```python
from build123d import *

# Parameters (mm, degrees)
SKETCH2_W                      = 45
SKETCH2_H                      = 24
BOSS_EXTRUDE1_DEPTH            = 50
CUT_EXTRUDE7_DEPTH             = 50
CHAMFER4_SIZE                  = 6
CUT_EXTRUDE1_REACH             = 70.33
SKETCH3_W                      = 45
SKETCH3_H                      = 10
CUT_EXTRUDE2_REACH             = 55.912
SKETCH4_R                      = 2
CUT_EXTRUDE2_DIRECTION_2_REACH = 55.912
SKETCH8_W                      = 45
SKETCH8_H                      = 50
CUT_EXTRUDE4_DEPTH             = 14
SKETCH6_R                      = 4
BOSS_EXTRUDE2_DEPTH            = 45
CUT_EXTRUDE3_START             = -50
SKETCH7_R                      = 2
CUT_EXTRUDE3_DEPTH             = 50
CUT_EXTRUDE6_START             = -2.5
SKETCH13_R                     = 2
CUT_EXTRUDE6_DEPTH             = 50
BOSS_EXTRUDE16_REACH           = 58.127
CUT_EXTRUDE13_REACH            = 64.292
SKETCH30_W                     = 45
SKETCH30_H                     = 10
CUT_EXTRUDE18_START            = -50
SKETCH37_R                     = 2
CUT_EXTRUDE18_DEPTH            = 50
CUT_EXTRUDE20_REACH            = 62.83
SKETCH43_R                     = 1.5
SKETCH44_R                     = 3.05
CUT_EXTRUDE21_DEPTH            = 1.1
SKETCH45_R                     = 3.05
CUT_EXTRUDE22_DEPTH            = 1.1
BOSS_EXTRUDE23_DEPTH           = 2.5
BOSS_EXTRUDE24_DEPTH           = 2.5
SKETCH55_R                     = 3.05
CUT_EXTRUDE28_DEPTH            = 1.1
CUT_EXTRUDE29_START            = -50
SKETCH57_R                     = 1.5
CUT_EXTRUDE29_DEPTH            = 48.9
SKETCH58_R                     = 3.05
CUT_EXTRUDE30_DEPTH            = 1.1
CHAMFER11_SIZE                 = 3
BOSS_EXTRUDE19_DEPTH           = 8
BOSS_EXTRUDE20_DEPTH           = 8
CHAMFER7_SIZE                  = 1
CHAMFER8_SIZE                  = 1


with BuildPart() as part:
    # Sketch2 → Boss-Extrude1 (new body)
    with BuildSketch(Plane(origin=(0, 0, 0), x_dir=(0, 0, -1), z_dir=(1, 0, 0))):
        Rectangle(SKETCH2_W, SKETCH2_H)
    extrude(amount=BOSS_EXTRUDE1_DEPTH)

    # Sketch14 → Cut-Extrude7 (cut)
    with BuildSketch(Plane(origin=(50, 0, 0), x_dir=(0, 0, -1), z_dir=(1, 0, 0))):
        Polygon((2.5, 12), (22.5, 2), (22.5, 12), align=None)
    extrude(amount=-CUT_EXTRUDE7_DEPTH, mode=Mode.SUBTRACT)

    # Chamfer4
    chamfer4_edges = [part.edges().sort_by_distance(p)[0] for p in [
        (25, -12, 22.5),
        (25, 12, 22.5),
    ]]
    chamfer(chamfer4_edges, length=CHAMFER4_SIZE)

    # Cut-Extrude1: up to this face of the body (flat: up to its plane)
    cut_extrude1_end = Plane(part.part.faces().sort_by_distance((25, 0, 22.5))[0])
    # Sketch3 → Cut-Extrude1 (cut, up to the picked face)
    with BuildSketch(Plane(origin=(0, 0, -22.5), x_dir=(-1, 0, 0), z_dir=(0, 0, -1)), mode=Mode.PRIVATE) as cut_extrude1_sk1:
        with Locations((-25, -7)):
            Rectangle(SKETCH3_W, SKETCH3_H)
    cut_extrude1_tool1 = split(extrude(cut_extrude1_sk1.sketch, amount=-CUT_EXTRUDE1_REACH, mode=Mode.PRIVATE), bisect_by=cut_extrude1_end, keep=Keep.BOTH, mode=Mode.PRIVATE)
    add(cut_extrude1_tool1.solids().sort_by(Axis((25, -7, -22.5), (0, 0, 1)))[0], mode=Mode.SUBTRACT)

    # Cut-Extrude2: up to this face of the body (flat: up to its plane)
    cut_extrude2_end = Plane(part.part.faces().sort_by_distance((50, -0.918079096, 0.895480226))[0])
    # Sketch4 → Cut-Extrude2 (cut, up to the picked face)
    with BuildSketch(Plane(origin=(2.5, 0, 0), x_dir=(0, 0, -1), z_dir=(1, 0, 0)), mode=Mode.PRIVATE) as cut_extrude2_sk1:
        with Locations(Location((14.5, -4, 0), (0, 0, 180))):
            Circle(SKETCH4_R)
    cut_extrude2_tool1 = split(extrude(cut_extrude2_sk1.sketch, amount=CUT_EXTRUDE2_REACH, mode=Mode.PRIVATE), bisect_by=cut_extrude2_end, keep=Keep.BOTH, mode=Mode.PRIVATE)
    add(cut_extrude2_tool1.solids().sort_by(Axis((2.5, -4, -14.5), (1, 0, 0)))[0], mode=Mode.SUBTRACT)

    # Cut-Extrude2 direction 2: up to this face of the body (flat: up to its plane)
    cut_extrude2_direction_2_end = Plane(part.part.faces().sort_by_distance((0, -0.918079096, 0.895480226))[0])
    # Sketch4 → Cut-Extrude2 direction 2 (cut, up to the picked face)
    with BuildSketch(Plane(origin=(2.5, 0, 0), x_dir=(0, 0, -1), z_dir=(1, 0, 0)), mode=Mode.PRIVATE) as cut_extrude2_direction_2_sk1:
        with Locations(Location((14.5, -4, 0), (0, 0, 180))):
            Circle(SKETCH4_R)
    cut_extrude2_direction_2_tool1 = split(extrude(cut_extrude2_direction_2_sk1.sketch, amount=-CUT_EXTRUDE2_DIRECTION_2_REACH, mode=Mode.PRIVATE), bisect_by=cut_extrude2_direction_2_end, keep=Keep.BOTH, mode=Mode.PRIVATE)
    add(cut_extrude2_direction_2_tool1.solids().sort_by(Axis((2.5, -4, -14.5), (-1, 0, 0)))[0], mode=Mode.SUBTRACT)

    # Sketch8 → Cut-Extrude4 (cut)
    with BuildSketch(Plane(origin=(0, 12, 0), x_dir=(1, 0, 0), z_dir=(0, 1, 0))):
        with Locations((25, 2.5)):
            Rectangle(SKETCH8_W, SKETCH8_H)
    extrude(amount=-CUT_EXTRUDE4_DEPTH, mode=Mode.SUBTRACT)


with BuildPart() as cut_extrude4_piece_1:
    # of the separate pieces the step leaves, piece 1, a body of its own (cut_extrude4_pieces)
    add(part.part.solids().sort_by_distance((0, -12, 16.5))[0])


with BuildPart() as cut_extrude4_piece_2:
    # of the separate pieces the step leaves, piece 2, a body of its own (cut_extrude4_pieces)
    add(part.part.solids().sort_by_distance((50, 2, -22.5))[0])

    # Sketch6 → Boss-Extrude2 (add)
    with BuildSketch(Plane(origin=(2.5, 0, 0), x_dir=(0, 0, -1), z_dir=(1, 0, 0))):
        with Locations(Location((14.5, -4, 0), (0, 0, 180))):
            Circle(SKETCH6_R)
    extrude(amount=BOSS_EXTRUDE2_DEPTH)


with BuildPart() as cut_extrude3_tool:
    # Sketch7 → Cut-Extrude3 (new body)
    with BuildSketch(Plane.ZY.offset(CUT_EXTRUDE3_START)):
        with Locations((11, 0)):
            Circle(SKETCH7_R)
    extrude(amount=CUT_EXTRUDE3_DEPTH)


with BuildPart() as cut_extrude4_piece_1_1:
    add(cut_extrude4_piece_1.part)

    # Cut-Extrude3: cut by cut_extrude3_tool
    add(cut_extrude3_tool.part, mode=Mode.SUBTRACT)


with BuildPart() as cut_extrude4_piece_2_1:
    add(cut_extrude4_piece_2.part)

    # Cut-Extrude3: cut by cut_extrude3_tool
    add(cut_extrude3_tool.part, mode=Mode.SUBTRACT)


with BuildPart() as cut_extrude6_tool:
    # Sketch13 → Cut-Extrude6 (new body)
    with BuildSketch(Plane.ZY.offset(-47.5).offset(CUT_EXTRUDE6_START)):
        with Locations(Location((-2.5, -4, 0), (0, 0, 270))):
            Circle(SKETCH13_R)
    extrude(amount=CUT_EXTRUDE6_DEPTH)


with BuildPart() as cut_extrude4_piece_1_2:
    add(cut_extrude4_piece_1_1.part)

    # Cut-Extrude6: cut by cut_extrude6_tool
    add(cut_extrude6_tool.part, mode=Mode.SUBTRACT)


with BuildPart() as cut_extrude4_piece_2_2:
    add(cut_extrude4_piece_2_1.part)

    # Cut-Extrude6: cut by cut_extrude6_tool
    add(cut_extrude6_tool.part, mode=Mode.SUBTRACT)

    # Boss-Extrude16: up to this face of the body (flat: up to its plane)
    boss_extrude16_end = Plane(cut_extrude4_piece_2_2.part.faces().sort_by_distance((50, -0.845343651, 1.015922603))[0])
    # Sketch29 → Boss-Extrude16 (add, up to the picked face)
    with BuildSketch(Plane.ZY, mode=Mode.PRIVATE) as boss_extrude16_sk1:
        Polygon((28.985281374, 6), (22.5, 6), (22.5, -6), (28.985281374, -6), (32.5, -2.485281374), (32.5, 2.485281374), align=None)
    boss_extrude16_tool1 = split(extrude(boss_extrude16_sk1.sketch, amount=-BOSS_EXTRUDE16_REACH, mode=Mode.PRIVATE), bisect_by=boss_extrude16_end, keep=Keep.BOTH, mode=Mode.PRIVATE)

    add(cut_extrude4_piece_1_2.part)  # Boss-Extrude16 merges Cut-Extrude4 piece 1
    add(boss_extrude16_tool1.solids().sort_by(Axis((0, 0, 27.06066), (1, 0, 0)))[0])

    # Cut-Extrude13: up to this plane
    cut_extrude13_end = Plane(origin=(65.620499352, -6, 28.985281374), z_dir=(0, -0.7071067811865474, 0.7071067811865477))
    # Sketch30 → Cut-Extrude13 (cut, up to the surface)
    with BuildSketch(Plane(origin=(0, 6, 0), x_dir=(1, 0, 0), z_dir=(0, 1, 0)), mode=Mode.PRIVATE) as cut_extrude13_sk1:
        with Locations((25, -27.5)):
            Rectangle(SKETCH30_W, SKETCH30_H)
    cut_extrude13_tool1 = split(extrude(cut_extrude13_sk1.sketch, amount=-CUT_EXTRUDE13_REACH, mode=Mode.PRIVATE), bisect_by=cut_extrude13_end, keep=Keep.BOTH, mode=Mode.PRIVATE)
    add(cut_extrude13_tool1.solids().sort_by_distance((25, 6, 27.5))[0], mode=Mode.SUBTRACT)

    # Sketch37 → Cut-Extrude18 (cut)
    with BuildSketch(Plane.ZY.offset(CUT_EXTRUDE18_START)):
        with Locations((27.5, 0)):
            Circle(SKETCH37_R)
    extrude(amount=CUT_EXTRUDE18_DEPTH, mode=Mode.SUBTRACT)

    # Cut-Extrude20: up to this face of the body (flat: up to its plane)
    cut_extrude20_end = Plane(cut_extrude4_piece_2_2.part.faces().sort_by_distance((0, -0.765078921, 3.483337135))[0])
    # Sketch43 → Cut-Extrude20 (cut, up to the picked face)
    with BuildSketch(Plane(origin=(50, 0, 0), x_dir=(0, 0, -1), z_dir=(1, 0, 0)), mode=Mode.PRIVATE) as cut_extrude20_sk1:
        with Locations((7.5, 3)):
            Circle(SKETCH43_R)
    cut_extrude20_tool1 = split(extrude(cut_extrude20_sk1.sketch, amount=-CUT_EXTRUDE20_REACH, mode=Mode.PRIVATE), bisect_by=cut_extrude20_end, keep=Keep.BOTH, mode=Mode.PRIVATE)
    add(cut_extrude20_tool1.solids().sort_by(Axis((50, 3, -7.5), (-1, 0, 0)))[0], mode=Mode.SUBTRACT)

    # Sketch44 → Cut-Extrude21 (cut)
    with BuildSketch(Plane(origin=(50, 0, 0), x_dir=(0, 0, -1), z_dir=(1, 0, 0))):
        with Locations((7.5, 3)):
            Circle(SKETCH44_R)
    extrude(amount=-CUT_EXTRUDE21_DEPTH, mode=Mode.SUBTRACT)

    # Sketch45 → Cut-Extrude22 (cut)
    with BuildSketch(Plane.ZY):
        with Locations(Location((-7.5, 3, 0), (0, 0, 180))):
            Circle(SKETCH45_R)
    extrude(amount=-CUT_EXTRUDE22_DEPTH, mode=Mode.SUBTRACT)

    # Sketch48 → Boss-Extrude23 (add)
    with BuildSketch(Plane(origin=(50, 0, 0), x_dir=(0, 0, -1), z_dir=(1, 0, 0))):
        Polygon((-16.5, 12), (-22.5, 6), (-28.985281374, 6), (-32.5, 2.485281374), (-32.5, 12), align=None)
    extrude(amount=-BOSS_EXTRUDE23_DEPTH)

    # Sketch49 → Boss-Extrude24 (add)
    with BuildSketch(Plane.ZY):
        Polygon((28.985281374, 6), (22.5, 6), (16.5, 12), (32.5, 12), (32.5, 2.485281374), align=None)
    extrude(amount=-BOSS_EXTRUDE24_DEPTH)

    # Sketch55 → Cut-Extrude28 (cut)
    with BuildSketch(Plane.ZY):
        with Locations((27.5, 7)):
            Circle(SKETCH55_R)
    extrude(amount=-CUT_EXTRUDE28_DEPTH, mode=Mode.SUBTRACT)

    # Sketch57 → Cut-Extrude29 (cut)
    with BuildSketch(Plane.ZY.offset(CUT_EXTRUDE29_START)):
        with Locations((27.5, 7)):
            Circle(SKETCH57_R)
    extrude(amount=CUT_EXTRUDE29_DEPTH, mode=Mode.SUBTRACT)

    # Sketch58 → Cut-Extrude30 (cut)
    with BuildSketch(Plane(origin=(50, 0, 0), x_dir=(0, 0, -1), z_dir=(1, 0, 0))):
        with Locations(Location((-27.5, 7, 0), (0, 0, 180))):
            Circle(SKETCH58_R)
    extrude(amount=-CUT_EXTRUDE30_DEPTH, mode=Mode.SUBTRACT)

    # Chamfer11
    chamfer11_edges = [cut_extrude4_piece_2_2.edges().sort_by_distance(p)[0] for p in [
        (48.75, 12, 32.5),
        (1.25, 12, 32.5),
    ]]
    chamfer(chamfer11_edges, length=CHAMFER11_SIZE)

    # Sketch38 → Boss-Extrude19 (add)
    with BuildSketch(Plane.ZY):
        Polygon((-2.5, 12), (-22.5, 2), (-22.5, -12), (16.5, -12), (22.5, -6), (22.5, 6), (16.5, 12), align=None)
    extrude(amount=BOSS_EXTRUDE19_DEPTH)

    # Sketch39 → Boss-Extrude20 (add)
    with BuildSketch(Plane(origin=(50, 0, 0), x_dir=(0, 0, -1), z_dir=(1, 0, 0))):
        Polygon((-22.5, 6), (-22.5, -6), (-16.5, -12), (22.5, -12), (22.5, 2), (2.5, 12), (-16.5, 12), align=None)
    extrude(amount=BOSS_EXTRUDE20_DEPTH)

    # Chamfer7
    chamfer7_edges = [cut_extrude4_piece_2_2.edges().sort_by_distance(p)[0] for p in [
        (-8, 12, 7),
        (-8, 7, -12.5),
        (-8, -5, -22.5),
        (-8, -12, -3),
        (-8, -9, 19.5),
        (-8, 0, 22.5),
        (-8, 9, 19.5),
        (58, 9, 19.5),
        (58, 0, 22.5),
        (58, -9, 19.5),
        (58, -12, -3),
        (58, -5, -22.5),
        (58, 7, -12.5),
        (58, 12, 7),
    ]]
    chamfer(chamfer7_edges, length=CHAMFER7_SIZE)

    # Chamfer8
    chamfer8_edges = [cut_extrude4_piece_2_2.edges().sort_by_distance(p)[0] for p in [
        (47.5, -12, -3),
        (47.5, -5, -22.5),
        (47.5, -9, 19.5),
        (47.5, 7, -12.5),
    ]]
    chamfer(chamfer8_edges, length=CHAMFER8_SIZE)


solid = cut_extrude4_piece_2_2.part
```
Model file for the job. Use its own axes, mm. A direction names the side the tool comes from. Coordinates: 2 decimals unless noted, no trailing zeros. Order: outer loops, then holes, each group sorted by start corner. A loop starts at its lowest first (then second) coordinate and runs counter-clockwise, first axis right, second up. Notation, with made-up numbers: (71.5, -32) -> (90.5, -32) arc R21 ccw to (90.5, -1) -> close; hole circle Ø9 at (23.5, -12). An arc over 180 degrees is marked (long way). Answer as a JSON object with one key per item and string values. Group by question number.
1) Drill centre lines: L1, parallel to X at y = 11.25, z = 20.5; L2, parallel to Y at x = 1.7, z = -2.5; L3, parallel to X at y = -2.5, z = 7. Where is each one in solid material? Low to high.
2) Flat gauge pins, fed straight in: pin 1 (3 mm diameter, centred on y = 0, z = 27.5, fed in from +X); pin 2 (13 mm diameter, centred on y = 4.5, z = 23, fed in from -X); pin 3 (4 mm diameter, centred on y = 7, z = 27.5, fed in from -X); pin 4 (2 mm diameter, centred on x = 52.5, y = 1, fed in from +Z). Where does each tip first touch, or does it go through?
3) Cut at A-A, the plane z = 11. Write the cut outline in (x, y).
4) Cut at B-B, the plane y = 7. Count the separate pieces of the cut face and the enclosed holes in it, then the cut area to 3 significant figures.
5) Which spindle directions (+Z, -Z, +X, -X, +Y, -Y) get a long thin tool onto all of the face, cutting with end or side? Do faces 1 (the face through (1.1, 4, -6)), 2 (the face through (-3.5, 9, 19.5)), 3 (the face through (53.5, 9, 19.5)), 4 (the face through (53, -5, -22.5)). Say none if no direction does.
6) Pull direction X, two halves, no side cores. Call faces 5 (the face through (50, 3, 26)), 6 (the face through (24.7, -1.6, -17.7)), 7 (the face through (-2, -12, -3)): +X half, -X half, draft (parallel to the pull), parting line (faces both ways), or undercut.
Check values:
{
 "1": {"L1": "x = 0 to 2.5, 47.5 to 50", "L2": "y = -12 to -6, -2 to 12", "L3": "x = -8 to 2.5, 47.5 to 58"},
 "2": {"pin 1": "passes through", "pin 2": "stops at x = -8", "pin 3": "stops at x = 1.1", "pin 4": "stops at z = 22.5"},
 "3": {"outline": "(-8, -11) -> (-7, -12) -> (2.5, -12) -> (2.5, -2) -> (0, -2) -> (0, 2) -> (2.5, 2) -> (2.5, 12) -> (-7, 12) -> (-8, 11) -> close; (47.5, -11) -> (48.5, -12) -> (57, -12) -> (58, -11) -> (58, 11) -> (57, 12) -> (47.5, 12) -> (47.5, 2) -> (50, 2) -> (50, -2) -> (47.5, -2) -> close"},
 "4": {"separate pieces": "4", "enclosed holes": "0", "area": "742 mm²"},
 "5": {"face 1": "none", "face 2": "+Z, -X, +Y", "face 3": "+Z, +X, +Y", "face 4": "-Z, +X, -X, +Y, -Y"},
 "6": {"face 5": "+X half", "face 6": "undercut", "face 7": "draft"}
}
